Build history of the part. All positions in model axes, mm. A direction names the side the tool comes from. Coordinates: 2 decimals unless noted, no trailing zeros. Order: outer loops, then holes, each group sorted by start corner. A loop starts at its lowest first (then second) coordinate and runs counter-clockwise, first axis right, second up. Notation, with made-up numbers: M -11,23 L 35,23 A29 ccw 35,53 Z; hole C -22.5,-10 d3. An arc over 180 degrees is marked long. Write item = value, one per line. Start each with the question number.
Q1. Drill centre lines: probe 1 along Y at (x, z) = (-15.5, 6); probe 2 along X at (y, z) = (-9.5, 2.25); probe 3 along Y at (x, z) = (11, 3.25). Where is each one in solid material? Low to high.
Q2. 3-axis set-ups, long thin cutter, end or side, ignore diameter. For faces 5 (the face through (7.541, -124, 3)), 6 (the face through (-12.541, -96, 3)), 7 (the face through (0, 120.703, 3)), 8 (the face through (0, -120.703, 3)), 9 (the face through (-10, 120.703, 3)): which of +Z, -Z, +X, -X, +Y, -Y reach the whole face in a straight line?
Q3. Pull direction X, two halves, no side cores. Call faces 1 (the face through (-16, 72.438, 3)), 2 (the face through (2.459, 124, 3)), 3 (the face through (27.541, -101, 3)), 4 (the face through (-2.459, -124, 3)): released by +X, released by -X, zero draft, split by the parting line, or undercut.
Q4. Band-saw the part on B-B on y = -100.5. Write the cut outline in (x, z).
Q5. Pin check, flat tips, straight feed: P1, Ø1.9, axis at y = -123, z = 4.5, coming from the +X side; P2, Ø3, axis at x = 26, z = 1, coming from the -Y side; P3, Ø1.9, axis at y = -10, z = 3, coming from the -X side. Stop position of each tip, or through.
Q6. Band-saw the part on C-C on x = 31.5. Write the cut outline in (y, z), plus the area to 3 significant figures.
```python
from build123d import *

# Parameters (mm, degrees)
SKETCH1_W           = 5
SKETCH1_H           = 6.35
SKETCH1_W_2         = 25
SKETCH1_H_2         = 241.325
SKETCH1_W_3         = 6.4
SKETCH1_H_3         = 48.265
SKETCH1_W_4         = 15
SKETCH1_W_5         = 12
SKETCH1_H_4         = 201.325
BOSS_EXTRUDE1_DEPTH = 6.35
BOSS_EXTRUDE2_DEPTH = 6.35


with BuildPart() as part:
    # Sketch1 → Boss-Extrude1 (new body)
    with BuildSketch(Plane.XY):
        with Locations((-5, 123.8375)):
            Rectangle(SKETCH1_W, SKETCH1_H)
        with Locations((5, 123.8375)):
            Rectangle(SKETCH1_W, SKETCH1_H)
        Rectangle(SKETCH1_W_2, SKETCH1_H_2)
        with Locations((-15.7, 48.265)):
            Rectangle(SKETCH1_W_3, SKETCH1_H_3)
        with Locations((-15.7, -48.265)):
            Rectangle(SKETCH1_W_3, SKETCH1_H_3)
        with Locations((-5, -123.8375)):
            Rectangle(SKETCH1_W, SKETCH1_H)
        with Locations((5, -123.8375)):
            Rectangle(SKETCH1_W, SKETCH1_H)
        with Locations((20, 0)):
            Rectangle(SKETCH1_W_4, SKETCH1_H_2)
        with Locations((33.5, 20)):
            Rectangle(SKETCH1_W_5, SKETCH1_H_4)
    extrude(amount=BOSS_EXTRUDE1_DEPTH)

    # Sketch2 → Boss-Extrude2 (add)
    with BuildSketch(Plane.XY.offset(6.35)):
        Polygon((27.54064, -120.70314), (27.54064, -80.70314), (39.54064, -80.70314), (39.54064, 120.70314), (7.54064, 120.70314), (7.54064, 127.05314), (2.45936, 127.05314), (2.45936, 120.70314), (-2.45936, 120.70314), (-2.45936, 127.05314), (-7.54064, 127.05314), (-7.54064, 120.70314), (-12.54064, 120.70314), (-12.54064, 72.43814), (-18.94064, 72.43814), (-18.94064, 24.09186), (-12.54064, 24.09186), (-12.54064, -24.09186), (-18.94064, -24.09186), (-18.94064, -72.43814), (-12.54064, -72.43814), (-12.54064, -120.70314), (-7.54064, -120.70314), (-7.54064, -127.05314), (-2.45936, -127.05314), (-2.45936, -120.70314), (2.45936, -120.70314), (2.45936, -127.05314), (7.54064, -127.05314), (7.54064, -120.70314), align=None)
    extrude(amount=-BOSS_EXTRUDE2_DEPTH)


solid = part.part
```
Recorded:
q1.probe_1 = -72.44 to -24.09, 24.09 to 72.44
q1.probe_2 = -12.54 to 39.54
q1.probe_3 = -120.7 to 120.7
q2.face_5 = +Z, -Z, +X, -Y
q2.face_6 = +Z, -Z, -X, -Y
q2.face_7 = +Z, -Z, +Y
q2.face_8 = +Z, -Z, -Y
q2.face_9 = +Z, -Z, -X, +Y
q3.face_1 = zero draft
q3.face_2 = undercut
q3.face_3 = released by +X
q3.face_4 = undercut
q4.outline = M -12.54,0 L 27.54,0 L 27.54,6.35 L -12.54,6.35 Z
q5.P1 = 7.54
q5.P2 = -120.7
q5.P3 = -12.54
q6.outline = M -80.7,0 L 120.7,0 L 120.7,6.35 L -80.7,6.35 Z
q6.area = 1,280 mm2
